```python
from build123d import *

# Parameters (mm, degrees)
F0_W     = 145.192
F0_H     = 91.725
F1_DEPTH = 3
F2_W     = 133.192
F2_H     = 79.725
F3_DEPTH = 3
F4_W     = 3
F4_H     = 20
F5_DEPTH = 16.5
F7_DEPTH = 20


with BuildPart() as f1:
    # F0 (on Top) → F1 (new body)
    with BuildSketch(Plane.XY):
        Rectangle(F0_W, F0_H)
    extrude(amount=F1_DEPTH)

    # F2 (on face) → F3 (cut)
    with BuildSketch(Plane.XY.offset(3)):
        Rectangle(F2_W, F2_H)
    extrude(amount=-F3_DEPTH, mode=Mode.SUBTRACT)

    # F4 (on face) → F5 (join)
    with BuildSketch(Plane.XY.offset(3)):
        with Locations((-71.096, 0)):
            Rectangle(F4_W, F4_H)
    extrude(amount=F5_DEPTH)

    # F6 (on face) → F7 (join)
    with BuildSketch(Plane.XZ.offset(10)):
        Polygon((-64.596, 19.5), (-69.596, 19.5), (-69.596, 11.3592599663), (-64.596, 18.5), align=None)
    extrude(amount=-F7_DEPTH)

    # F8: F1 across plane


with BuildPart() as f1_1:
    add(f1.part)
    add(f1.part.mirror(Plane.YZ))


solid = f1_1.part
```
Design review of the part built by this model. Coordinates are the model's own, in mm. A direction names the side the tool comes from. Round coordinates to 2 decimals unless told otherwise and drop trailing zeros. Order: outer loops, then holes, each group sorted by start corner. A loop starts at its lowest first (then second) coordinate and runs counter-clockwise, first axis right, second up. Notation, with made-up numbers: (18.5, 20) - (38.5, 20) arc R13 cw to (38.5, 25) - close; hole circle Ø4 at (39, -11). An arc over 180 degrees is marked (long way). One line per question, with ' | ' between items.
Item 1: Take a section at B-B, the plane z = 5.75. Write out the cut boundary in (x, y).
Checks:
outline: (-72.6, -10) - (-69.6, -10) - (-69.6, 10) - (-72.6, 10) - close; (69.6, -10) - (72.6, -10) - (72.6, 10) - (69.6, 10) - close
Item 2: Machinability: for faces 1 (the face through (-66.596, -1, 2)), 2 (the face through (70, 10, 13)), 3 (the face through (70, -10, 13)), 4 (the face through (-1, 39.862, 2)), 5 (the face through (-69.596, 0, 7)), which of the approach directions +Z, -Z, +X, -X, +Y, -Y give a long, thin tool a straight path to every point of the face, cutting with its end or side? Answer none if there is none.
Checks:
face 1: -Z | face 2: +Z, +X, -X, +Y | face 3: +Z, +X, -X, -Y | face 4: +Z, -Z | face 5: +Y, -Y
Item 3: Draft analysis for pull direction X (two halves, no side actions). For faces 6 (the face through (-70, -10, 13)), 7 (the face through (66.596, -1, 2)), 8 (the face through (-72.596, 0, 7)), state which applies: +X half, -X half, draft (parallel to the pull), parting line (faces both ways), or undercut.
Checks:
face 6: draft | face 7: undercut | face 8: -X half
Item 4: Wall thickness on line 1 (X direction, y = -23, z = 1); line 2 (Y direction, x = 27, z = 1.75); line 3 (X direction, y = 7.5, z = 4.5): over which ranges is each line inside the solid? List them lowest first. Write a range as [from, to].
Checks:
line 1: [-72.6, -66.6], [66.6, 72.6] | line 2: [-45.86, -39.86], [39.86, 45.86] | line 3: [-72.6, -69.6], [69.6, 72.6]
Item 5: For P1, Ø9, axis at x = 69, z = 8, coming from the -Y side; P2, Ø2.5, axis at x = -67.5, z = 7.5, coming from the +Y side; P3, Ø2.5, axis at x = 70, z = 8, coming from the +Y side, all flat-tipped, find the tip position at first contact; note any pin that passes through.
Checks:
P1: y = -10 | P2: through | P3: y = 10
Item 6: Take a section at C-C, the plane y = -8. Write out the cut boundary in (x, z).
Checks:
outline: (-72.6, 0) - (-66.6, 0) - (-66.6, 3) - (-69.6, 3) - (-69.6, 11.36) - (-64.6, 18.5) - (-64.6, 19.5) - (-72.6, 19.5) - close; (64.6, 18.5) - (69.6, 11.36) - (69.6, 3) - (66.6, 3) - (66.6, 0) - (72.6, 0) - (72.6, 19.5) - (64.6, 19.5) - close
Item 7: Take a section at A-A, the plane y = 22. Write out the cut boundary in (x, z).
Checks:
outline: (-72.6, 0) - (-66.6, 0) - (-66.6, 3) - (-72.6, 3) - close; (66.6, 0) - (72.6, 0) - (72.6, 3) - (66.6, 3) - close
